from build123d import *

# Parameters (mm, degrees)
SKETCH1_W           = 596.9
SKETCH1_H           = 22.86
BOSS_EXTRUDE1_DEPTH = 3.175
SKETCH5_W           = 38.1
SKETCH5_H           = 3.429
CUT_EXTRUDE2_DEPTH  = 299.685667592
FILLET1_R           = 6.35


with BuildPart() as part:
    # Sketch1 → Boss-Extrude1 (new body)
    with BuildSketch(Plane(origin=(0, 0, 0), x_dir=(1, 0, 0), z_dir=(0, 1, 0))):
        Rectangle(SKETCH1_W, SKETCH1_H)
    extrude(amount=BOSS_EXTRUDE1_DEPTH)

    # Sketch5 → Cut-Extrude2 (cut, through all)
    with BuildSketch(Plane(origin=(0, 3.175, 0), x_dir=(1, 0, 0), z_dir=(0, 1, 0))):
        with Locations((-198.966666582, 0)):
            Rectangle(SKETCH5_W, SKETCH5_H)
        with Locations((-99.483333164, 0)):
            Rectangle(SKETCH5_W, SKETCH5_H)
        with Locations((1.69e-07, 0)):
            Rectangle(SKETCH5_W, SKETCH5_H)
        with Locations((99.483333333, 0)):
            Rectangle(SKETCH5_W, SKETCH5_H)
        with Locations((198.966666667, 0)):
            Rectangle(SKETCH5_W, SKETCH5_H)
    extrude(amount=-CUT_EXTRUDE2_DEPTH, mode=Mode.SUBTRACT)

    # Fillet1
    fillet1_edges = [part.edges().sort_by_distance(p)[0] for p in [
        (-298.45, 1.5875, -11.43),
        (298.45, 1.5875, -11.43),
        (298.45, 1.5875, 11.43),
        (-298.45, 1.5875, 11.43),
    ]]
    fillet(fillet1_edges, radius=FILLET1_R)


solid = part.part
Build history of the part. All positions in model axes, mm. Round coordinates to 2 decimals unless told otherwise and drop trailing zeros. Loops run counter-clockwise (first coordinate to the right, second up) from the corner with the lowest first, then second, coordinate; pieces in that order, holes last. Notation, with made-up numbers: (53.25, 30.5) -> (112.25, 30.5) arc R19 cw to (112.25, 51.5) -> close; hole circle Ø8 at (-18.75, 63). An arc over 180 degrees is marked (long way). One line per item, written item: value. Start each with the question number.
Q1. Cut at B-B on y = 2.4. List the corners of the cut face in (x, z).
Q2. Cut at A-A on x = -112. List the corners of the cut face in (y, z) (1 decimal).
Q3. Probe line 1 along X through (y, z) = (1.25, -0.5); line 2 along Z through (x, y) = (84, 2.1); line 3 along X through (y, z) = (2, -9). List the from-to ranges inside material, lowest first.
Computed:
1. outline: (-298.45, -5.08) arc R6.35 ccw to (-292.1, -11.43) -> (292.1, -11.43) arc R6.35 ccw to (298.45, -5.08) -> (298.45, 5.08) arc R6.35 ccw to (292.1, 11.43) -> (-292.1, 11.43) arc R6.35 ccw to (-298.45, 5.08) -> close; hole (-218.02, -1.71) -> (-179.92, -1.71) -> (-179.92, 1.71) -> (-218.02, 1.71) -> close; hole (-118.53, -1.71) -> (-80.43, -1.71) -> (-80.43, 1.71) -> (-118.53, 1.71) -> close; hole (-19.05, -1.71) -> (19.05, -1.71) -> (19.05, 1.71) -> (-19.05, 1.71) -> close; hole (80.43, -1.71) -> (118.53, -1.71) -> (118.53, 1.71) -> (80.43, 1.71) -> close; hole (179.92, -1.71) -> (218.02, -1.71) -> (218.02, 1.71) -> (179.92, 1.71) -> close
2. outline: (0, -11.4) -> (3.2, -11.4) -> (3.2, -1.7) -> (0, -1.7) -> close; (0, 1.7) -> (3.2, 1.7) -> (3.2, 11.4) -> (0, 11.4) -> close
3. line 1: -298.45 to -218.02, -179.92 to -118.53, -80.43 to -19.05, 19.05 to 80.43, 118.53 to 179.92, 218.02 to 298.45
3. line 2: -11.43 to -1.71, 1.71 to 11.43
3. line 3: -297.1 to 297.1
